from build123d import *

# Parameters (mm, degrees)
SKETCH1_R              = 5
BOSS_EXTRUDE1_DEPTH    = 62
SKETCH7_R              = 2.5
CUT_EXTRUDE1_DEPTH     = 26
M3_TAPPED_HOLE1_REACH  = 61.068
M3_TAPPED_HOLE1_BORE_R = 1.25
M3_TAPPED_HOLE2_REACH  = 61.068
M3_TAPPED_HOLE2_BORE_R = 1.25


with BuildPart() as part:
    # Sketch1 → Boss-Extrude1 (new body)
    with BuildSketch(Plane(origin=(0, 0, 0), x_dir=(1, 0, 0), z_dir=(0, 1, 0))):
        with Locations(Location((0, 0, 0), (0, 0, 270))):
            Circle(SKETCH1_R)
    extrude(amount=BOSS_EXTRUDE1_DEPTH)

    # Sketch7 → Cut-Extrude1 (cut)
    with BuildSketch(Plane(origin=(0, 62, 0), x_dir=(1, 0, 0), z_dir=(0, 1, 0))):
        with Locations(Location((0, 0, 0), (0, 0, 270))):
            Circle(SKETCH7_R)
    extrude(amount=-CUT_EXTRUDE1_DEPTH, mode=Mode.SUBTRACT)

    # M3 Tapped Hole1 bore (on position points) → M3 Tapped Hole1 (cut, up to next)
    with BuildSketch(Plane(origin=(0, 58, 5), x_dir=(1, 0, 0), z_dir=(0, 0, 1)), mode=Mode.PRIVATE) as m3_tapped_hole1_sk1:
        Circle(M3_TAPPED_HOLE1_BORE_R)
    m3_tapped_hole1_tool1 = extrude(m3_tapped_hole1_sk1.sketch, amount=-M3_TAPPED_HOLE1_REACH, mode=Mode.PRIVATE) & part.part
    add(m3_tapped_hole1_tool1.solids().sort_by_distance((0, 58, 5))[0], mode=Mode.SUBTRACT)

    # M3 Tapped Hole2 bore (on position points) → M3 Tapped Hole2 (cut, up to next)
    with BuildSketch(Plane(origin=(5, 58, 0), x_dir=(0, 0, 1), z_dir=(1, 0, 0)), mode=Mode.PRIVATE) as m3_tapped_hole2_sk1:
        Circle(M3_TAPPED_HOLE2_BORE_R)
    m3_tapped_hole2_tool1 = extrude(m3_tapped_hole2_sk1.sketch, amount=-M3_TAPPED_HOLE2_REACH, mode=Mode.PRIVATE) & part.part
    add(m3_tapped_hole2_tool1.solids().sort_by_distance((5, 58, 0))[0], mode=Mode.SUBTRACT)


solid = part.part
Check sheet for the modelled part. Datum: model origin and axes. Units: mm. A direction names the side the tool comes from. Round coordinates to 2 decimals unless told otherwise and drop trailing zeros. Loops run counter-clockwise (first coordinate to the right, second up) from the corner with the lowest first, then second, coordinate; pieces in that order, holes last. Notation, with made-up numbers: M 31.5,7 L 74.5,7 A8 ccw 74.5,18 Z; hole C 38,31.25 d11. An arc over 180 degrees is marked long. One line per question, with ' | ' between items. Start each with the question number.
Item 1: Section check C-C (y = 58). Record the boundary of the cut face in (x, z), and give its area (3 significant figures).
Item 2: Section check B-B (z = 0). Record the boundary of the cut face in (x, y).
Item 3: Gauge pin test, flat ends, axial feed: pin 1 Ø4 at (x, y) = (-2.5, 29.5) entering from -Z; pin 2 Ø3 at (x, y) = (3.5, 46.5) entering from +Z; pin 3 Ø2 at (y, z) = (42, -3) entering from -X. Record the tip position at first contact, or that the pin passes through.
Item 4: Release check for a two-part mould opening along Y. For faces 3 (the face through (0, 0, 0)), 4 (the face through (0, 36, 0)), 5 (the face through (3.6, 58.76, -0.99)), 6 (the face through (-0.99, 57.24, 3.6)) record: released by +Y, released by -Y, zero draft, split by the parting line, or undercut.
Item 5: Section check A-A (x = 0). Record the boundary of the cut face in (y, z).
Item 6: Set-up check for faces 1 (the face through (-1.5, 49.2, -2)), 2 (the face through (-4.88, 30.57, -1.08)): record each of +Z, -Z, +X, -X, +Y, -Y from which the full face is reachable in a straight line by a thin tool's end or side.
Item 7: Scan lines: probe 1 along X at (y, z) = (55, 0.25); probe 2 along Y at (x, z) = (3, 0); probe 3 along Y at (x, z) = (-1.75, -0.5). Record each from-to range of solid material in increasing order.
Item 8: Section check D-D (z = -4). Record the boundary of the cut face in (x, y), and give its area (3 significant figures).
Worked out:
1) outline: M -1.25,2.17 L -1.25,4.84 A5 ccw long 4.84,-1.25 L 2.17,-1.25 A2.5 cw long Z; M 1.25,2.17 A2.5 cw 2.17,1.25 L 4.84,1.25 A5 ccw 1.25,4.84 Z | area: 46.1 mm^2
2) outline: M -5,0 L 5,0 L 5,56.75 L 2.5,56.75 L 2.5,36 L -2.5,36 L -2.5,62 L -5,62 Z; M 2.5,59.25 L 5,59.25 L 5,62 L 2.5,62 Z
3) pin 1: z = -4.97 | pin 2: z = 4.58 | pin 3: x = -4.58
4) face 3: released by -Y | face 4: released by +Y | face 5: undercut | face 6: undercut
5) outline: M 0,-5 L 62,-5 L 62,-2.5 L 36,-2.5 L 36,2.5 L 56.75,2.5 L 56.75,5 L 0,5 Z; M 59.25,2.5 L 62,2.5 L 62,5 L 59.25,5 Z
6) face 1: +Y | face 2: +Y, -Y
7) probe 1: -4.99 to -2.49, 2.49 to 4.99 | probe 2: 0 to 56.75, 59.25 to 62 | probe 3: 0 to 36
8) outline: M -3,0 L 3,0 L 3,62 L -3,62 Z | area: 372 mm^2
